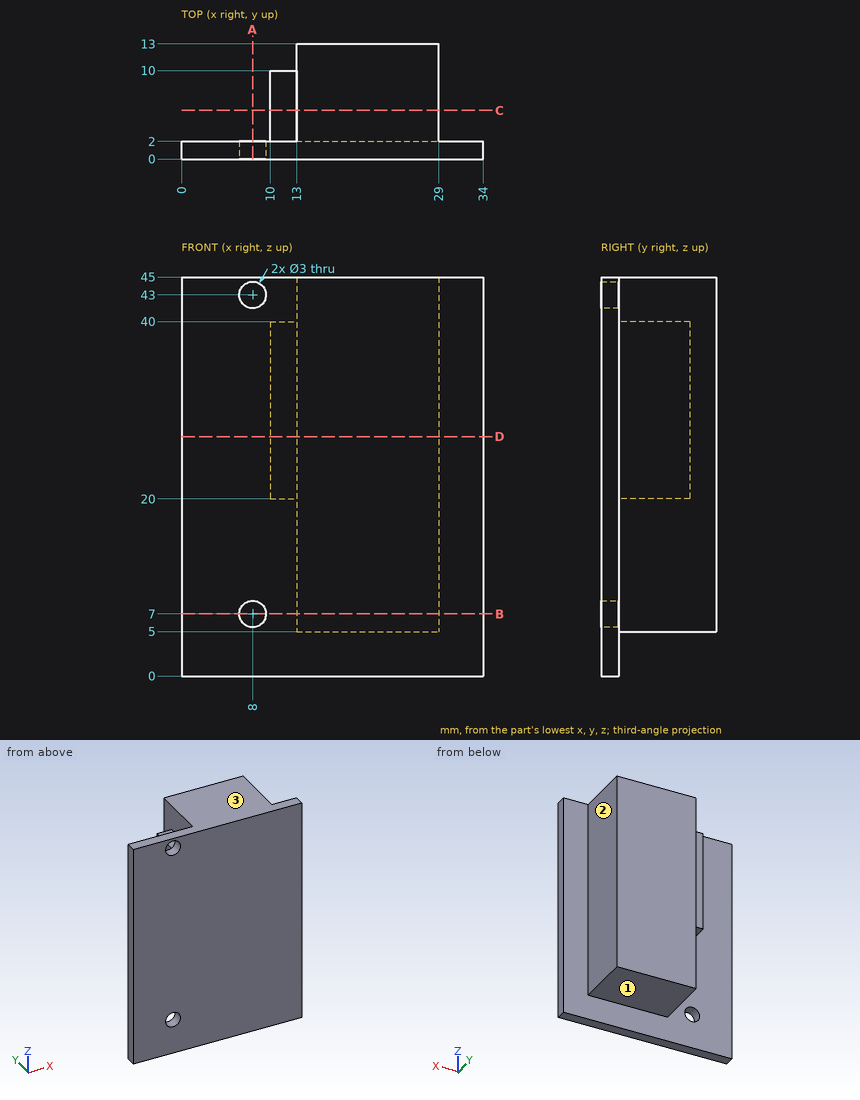
Geometry check sheet. Reference: drawing and pictorial views, mm from the part's lowest x, y, z. A direction names the side the tool comes from. Round coordinates to 2 decimals unless told otherwise and drop trailing zeros. Loops run counter-clockwise (first coordinate to the right, second up) from the corner with the lowest first, then second, coordinate; pieces in that order, holes last. Notation, with made-up numbers: (-2, 19) - (33, 19) arc R25 ccw to (33, 49) - close; hole circle Ø4 at (48.5, -18.75). An arc over 180 degrees is marked (long way). Answer in a Markdown table with one row per item. Add a question column.
Q1. Gauge pin test, flat ends, axial feed: pin 1 (1 mm diameter, centred on x = 4.5, z = 40, fed in from +Y); pin 2 (0.9 mm diameter, centred on x = 12, z = 33.5, fed in from +Y); pin 3 (2.5 mm diameter, centred on x = 11.5, y = 6.5, fed in from -Z). Record the tip position at first contact, or that the pin passes through.
Q2. Material ranges on line 1 (X direction, y = 1.5, z = 7); line 2 (Y direction, x = 32, z = 31.5); line 3 (X direction, y = 4.25, z = 38), recorded low to high.
Q3. Tool access check on the marked faces 1, 2 and 3. Record the directions out of +Z, -Z, +X, -X, +Y, -Y that give a thin tool (end or side, any length) a straight path to the whole face; none if there is none.
Q4. Section check C-C on y = 5.5. Enter the section's corners in (x, z).
Q5. Section check D-D on z = 27. Enter the section's corners in (x, y), plus the area to 3 significant figures.
Q6. Section check A-A on x = 8. Enter the section's corners in (y, z), plus the area to 3 significant figures.
Q7. Section check B-B on z = 7. Enter the section's corners in (x, y).
Found:
| question | item | result |
|---|---|---|
| 1 | pin 1 | stops at y = 2 |
| 1 | pin 2 | stops at y = 10 |
| 1 | pin 3 | stops at z = 20 |
| 2 | line 1 | x = 0 to 6.5, 9.5 to 34 |
| 2 | line 2 | y = 0 to 2 |
| 2 | line 3 | x = 10 to 29 |
| 3 | face 1 | -Z, +X, -X, +Y |
| 3 | face 2 | +Z, -Z, +X, +Y |
| 3 | face 3 | +Z, +X, -X, +Y, -Y |
| 4 | outline | (10, 20) - (13, 20) - (13, 5) - (29, 5) - (29, 45) - (13, 45) - (13, 40) - (10, 40) - close |
| 5 | outline | (0, 0) - (34, 0) - (34, 2) - (29, 2) - (29, 13) - (13, 13) - (13, 10) - (10, 10) - (10, 2) - (0, 2) - close |
| 5 | area | 268 mm² |
| 6 | outline | (0, 0) - (2, 0) - (2, 5.5) - (0, 5.5) - close; (0, 8.5) - (2, 8.5) - (2, 41.5) - (0, 41.5) - close; (0, 44.5) - (2, 44.5) - (2, 45) - (0, 45) - close |
| 6 | area | 78.0 mm² |
| 7 | outline | (0, 0) - (6.5, 0) - (6.5, 2) - (0, 2) - close; (9.5, 0) - (34, 0) - (34, 2) - (29, 2) - (29, 13) - (13, 13) - (13, 2) - (9.5, 2) - close |
